```python
from build123d import *

# Parameters (mm, degrees)
F0_R      = 6
F0_R_2    = 5.5
F1_DEPTH  = 465
F2_R      = 2.4414340199
F3_DEPTH  = 20
F5_D      = 8
F5_DEPTH  = 6.0010001
F6_D      = 8
F7_DEPTH  = 130
F7_FACE_R = 4.25
F8_DEPTH  = 240


with BuildPart() as f1:
    # F0 (on Top) → F1 (new body)
    with BuildSketch(Plane.XY):
        Circle(F0_R)
        Circle(F0_R_2, mode=Mode.SUBTRACT)
    extrude(amount=F1_DEPTH)

    # F2 (on Right) → F3 (join)
    with BuildSketch(Plane.YZ):
        with Locations((0, 25.2948626876)):
            Circle(F2_R)
    extrude(amount=F3_DEPTH)

    # F5 (through all, one way)
    with BuildSketch(Plane.YZ):
        with Locations((0, 15)):
            Circle(F5_D / 2)
    extrude(amount=-F5_DEPTH, mode=Mode.SUBTRACT)

    # F6 (through all)
    with Locations(Plane(origin=(0, 0, 0), x_dir=(0, 1, 0), z_dir=(-1, 0, 0))):
        with Locations((0, -15)):
            Hole(F6_D / 2)

    # F4 (on Right) → F7 (join, symmetric)
    with BuildSketch(Plane.YZ):
        with BuildLine():
            ThreePointArc((0, 10.75), (3.00520382, 11.99479618), (4.25, 15))
            ThreePointArc((4.25, 15), (-3.00520382, 18.00520382), (0, 10.75))
        make_face()
    extrude(amount=F7_DEPTH, both=True)

    # F7_face (on face) → F8 (join)
    with BuildSketch(Plane(origin=(130, 0, 15), x_dir=(0, 1, 0), z_dir=(1, 0, 0))):
        Circle(F7_FACE_R)
    extrude(amount=F8_DEPTH)


solid = f1.part
```
For this review, take the finished solid that the model builds, in its own axes (mm). Give positions to 0.01 mm unless a question says otherwise; leave off trailing zeros. Write each loop counter-clockwise with the first axis right and the second up, starting at its lowest first coordinate (ties: lowest second). Pieces come first, ordered by that corner, then holes. Notation, with made-up numbers: M 36,49.25 L 93,49.25 A34 cw 93,87.25 Z; hole C 75.5,63 d1. An arc over 180 degrees is marked long. One line per item, written item: value.
1) For line 1 (X direction, y = -0.75, z = 429); line 2 (X direction, y = 0, z = 115), list the stretches that pass through material, from the lowest coordinate up. Write a range as from..to.
Results are:
line 1: x = -5.95..-5.45, 5.45..5.95
line 2: x = -6..-5.5, 5.5..6
2) For P1, Ø1.5, axis at y = 0.5, z = 24.5, coming from the +X side; P2, Ø2.5, axis at y = 1, z = 24, coming from the -X side; P3, Ø2, axis at x = -51.5, y = 1, coming from the +Z side, all flat-tipped, find the tip position at first contact; note any pin that passes through.
Results are:
P1: stops at x = 20
P2: stops at x = -6
P3: stops at z = 19.25
3) Take a section at A-A, the plane z = 281. Write out the cut boundary in (x, y).
Results are:
outline: C 0,0 d12; hole C 0,0 d11
4) The part is to be moulded in two halves that separate along X. For faces 1 (the cylindrical face through (-6, 0, 229)), 2 (the cylindrical face through (-1.19, -5.37, 229.24)), 3 (the flat face through (3, -5, 465)), say which applies: +X half, -X half, draft (parallel to the pull), parting line (faces both ways), or undercut.
Results are:
face 1: parting line
face 2: undercut
face 3: draft
5) Take a section at B-B, the plane x = 304. Write out the cut boundary in (y, z).
Results are:
outline: C 0,15 d8.5
